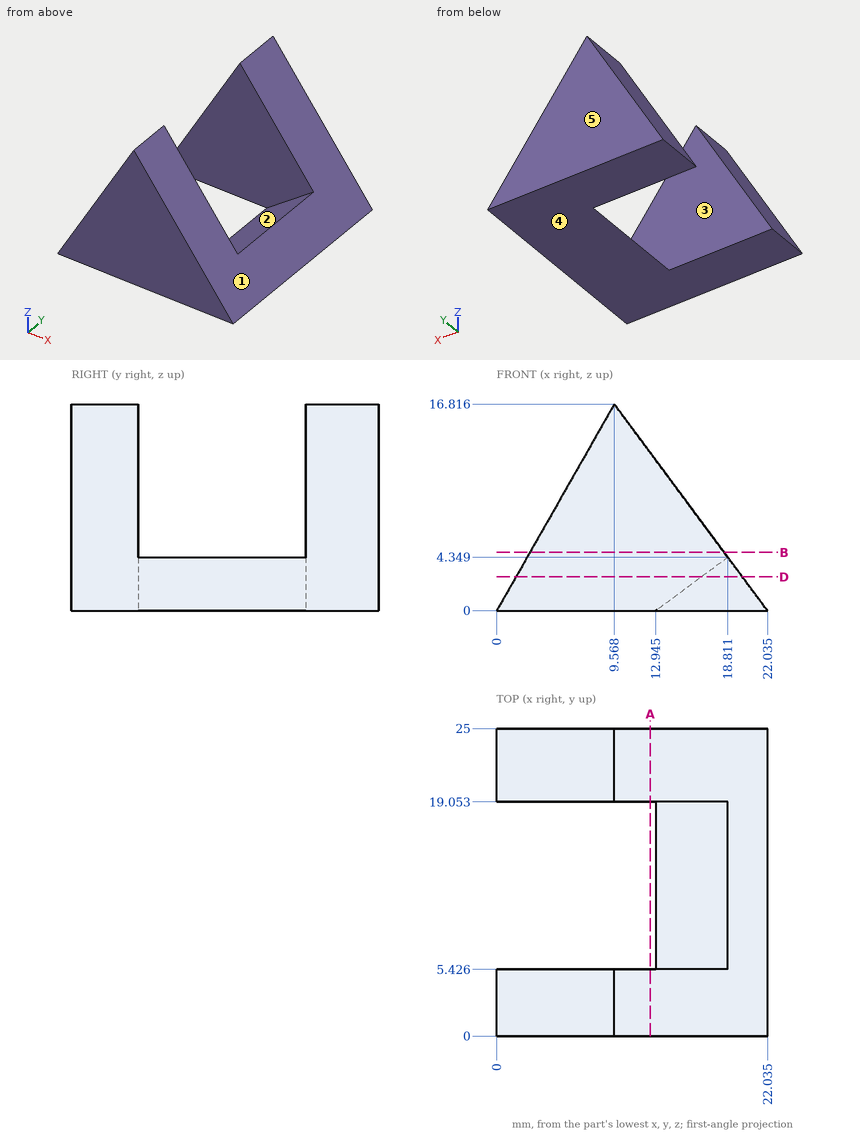
Can you work these out from the drawing? Everything is in mm from the part's minimum corner. A direction names the side the tool comes from. Round coordinates to 2 decimals unless told otherwise and drop trailing zeros. Order: outer loops, then holes, each group sorted by start corner. A loop starts at its lowest first (then second) coordinate and runs counter-clockwise, first axis right, second up. Notation, with made-up numbers: M 9,4 L 57,4 A29 cw 57,43 Z; hole C 75,24.5 d7. An arc over 180 degrees is marked long. Answer as CSV lines item,"result".
Item 1: Please list where these lines run through material, in increasing order: L1, parallel to Y at x = 14.25, z = 8.75 (1 decimal); L2, parallel to X at y = 2, z = 5.75; L3, parallel to Z at x = 16.25, y = 9.25. Write a range as [from, to].
From the geometry:
L1,"[0, 5.4], [19.1, 25]"
L2,"[3.27, 17.77]"
L3,"[0, 2.45]"
Item 2: We'd pull the mould along Y, two halves only. Please class the marked faces 3, 4 and 5: +Y half, -Y half, draft (parallel to the pull), parting line (faces both ways), or undercut.
From the geometry:
face 3,"undercut"
face 4,"draft"
face 5,"+Y half"
Item 3: Imagine slicing it at D-D on z = 2.75. List the corners of the cut face in (x, y) for me (1 decimal).
From the geometry:
outline,"M 1.6,0 L 20,0 L 20,25 L 1.6,25 L 1.6,19.1 L 16.7,19.1 L 16.7,5.4 L 1.6,5.4 Z"
Item 4: Imagine slicing it at B-B on z = 4.75. List the corners of the cut face in (x, y) for me (1 decimal), and give its area (3 significant figures).
From the geometry:
outline,"M 2.7,0 L 18.5,0 L 18.5,5.4 L 2.7,5.4 Z; M 2.7,19.1 L 18.5,19.1 L 18.5,25 L 2.7,25 Z"
area,"180 mm2"
Item 5: Imagine slicing it at A-A on x = 12.5. List the corners of the cut face in (y, z) for me (1 decimal), and give its area (3 significant figures).
From the geometry:
outline,"M 0,0 L 5.4,0 L 5.4,12.9 L 0,12.9 Z; M 19.1,0 L 25,0 L 25,12.9 L 19.1,12.9 Z"
area,"146 mm2"
Item 6: Which directions (+Z, -Z, +X, -X, +Y, -Y) give clear straight access to the entire face, cutting with the end or side of a thin tool? Please do the marked faces 1 and 2.
From the geometry:
face 1,"+Z, +X, +Y, -Y"
face 2,"+Z, -X"
Item 7: For pin 1 (1.5 mm diameter, centred on y = 4.5, z = 13, fed in from -X); pin 2 (3 mm diameter, centred on y = 20, z = 2, fed in from +X) (1 decimal); pin 3 (4 mm diameter, centred on y = 2.5, z = 7, fed in from -X) (1 decimal); pin 4 (8 mm diameter, centred on y = 14.5, z = 13.5, fed in from +X), each with a flat end and sliding along its axis, tell me the tip position at first contact or that it passes through.
From the geometry:
pin 1,"x = 6.97"
pin 2,"x = 21.7"
pin 3,"x = 2.8"
pin 4,"through"
